Here's how the part is built. I have some questions about the finished solid (model axes, mm). Face numbers are marked on the shaded views. A direction names the side the tool comes from. Give positions to 0.01 mm unless a question says otherwise; leave off trailing zeros. Loops run counter-clockwise (first coordinate to the right, second up) from the corner with the lowest first, then second, coordinate; pieces in that order, holes last.
Q1. Suppose I cut it at A-A (z = 25.2). List the corners of the cut face in (x, y) for me, and give its area (3 significant figures).
Q2. Suppose I cut it at D-D (x = -8.25). List the corners of the cut face in (y, z) for me.
Q3. I'm going to push flat-ended pins straight in: P1, Ø5, axis at x = 12.5, y = -3, coming from the +Z side; P2, Ø3.5, axis at x = 10, y = 0.5, coming from the -Z side; P3, Ø4, axis at y = -4.5, z = 1, coming from the +X side. Where does each tip first touch, or does it pass through?
Q4. Suppose I cut it at B-B (x = 6.5). List the corners of the cut face in (y, z) for me.
Q5. For the marked faces 1, 2 and 3, which set-ups out of +Z, -Z, +X, -X, +Y, -Y let a thin tool reach every point of the face, with its end or its side?
Q6. I need wall thicknesses on probe 1 along Z at (x, y) = (7.3, 0); probe 2 along Z at (x, y) = (-5.75, 2); probe 3 along X at (y, z) = (-4, -2). Which ranges of each line are inside material? Lowest first, please.
Q7. Suppose I cut it at C-C (y = -4.5). List the corners of the cut face in (x, z) for me.
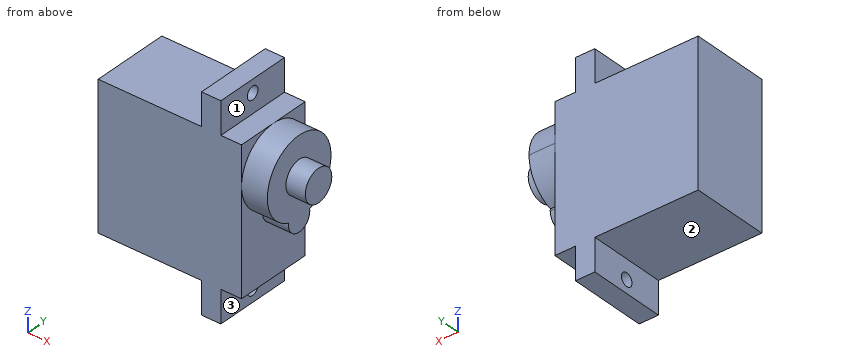
```python
from build123d import *

# Parameters (mm, degrees)
F1_DEPTH  = 22.2
F2_W      = 3
F2_H      = 12
F3_DEPTH  = 5
F4_W      = 3
F4_H      = 12
F5_DEPTH  = 5
F7_DEPTH  = 4
F8_R      = 2.5
F9_DEPTH  = 3
F10_R     = 1
F11_DEPTH = 25


with BuildPart() as f1:
    # F0 (on Top) → F1 (new body)
    with BuildSketch(Plane.XY):
        Polygon((-11.1, 6), (-11.1, 0), (-11.1, -6), (11.1, -6), (11.1, 0), (11.1, 6), align=None)
    extrude(amount=F1_DEPTH)

    # F2 (on face) → F3 (join)
    with BuildSketch(Plane.XY.offset(22.2)):
        with Locations((6.4, 0)):
            Rectangle(F2_W, F2_H)
    extrude(amount=F3_DEPTH)

    # F4 (on face) → F5 (join)
    with BuildSketch(Plane(origin=(0, 0, 0), x_dir=(1, 0, 0), z_dir=(0, 0, -1))):
        with Locations((6.4, 0)):
            Rectangle(F4_W, F4_H)
    extrude(amount=F5_DEPTH)

    # F6 (on face) → F7 (join)
    with BuildSketch(Plane.YZ.offset(11.1)):
        with BuildLine():
            ThreePointArc((1.9720265944, 10.5333333333), (4.8904069139, 12.7238066485), (6, 16.2))
            ThreePointArc((6, 16.2), (-3.4761933515, 21.0904069139), (-1.9720265944, 10.5333333333))
            ThreePointArc((-1.9720265944, 10.5333333333), (0, 12.2), (1.9720265944, 10.5333333333))
        make_face()
        with BuildLine():
            ThreePointArc((1.9720265944, 10.5333333333), (0, 12.2), (-1.9720265944, 10.5333333333))
            ThreePointArc((-1.9720265944, 10.5333333333), (0, 10.2), (1.9720265944, 10.5333333333))
        make_face()
        with BuildLine():
            ThreePointArc((1.9720265944, 10.5333333333), (0, 10.2), (-1.9720265944, 10.5333333333))
            ThreePointArc((-1.9720265944, 10.5333333333), (-0.1672525206, 8.2070056211), (2, 10.2))
            ThreePointArc((2, 10.2), (1.9929943789, 10.3672525206), (1.9720265944, 10.5333333333))
        make_face()
    extrude(amount=F7_DEPTH)

    # F8 (on face) → F9 (join)
    with BuildSketch(Plane.YZ.offset(15.1)):
        with Locations((0, 16.2)):
            Circle(F8_R)
    extrude(amount=F9_DEPTH)

    # F10 (on face) → F11 (cut)
    with BuildSketch(Plane(origin=(4.9, 0, 0), x_dir=(0, -1, 0), z_dir=(-1, 0, 0))):
        with Locations((0, 25.2)):
            Circle(F10_R)
        with Locations((0, -3)):
            Circle(F10_R)
    extrude(amount=-F11_DEPTH, mode=Mode.SUBTRACT)


solid = f1.part
```
Solutions:
1. outline: (4.9, -6) - (7.9, -6) - (7.9, -1) - (4.9, -1) - close; (4.9, 1) - (7.9, 1) - (7.9, 6) - (4.9, 6) - close
1. area: 30.0 mm2
2. outline: (-6, 0) - (6, 0) - (6, 22.2) - (-6, 22.2) - close
3. P1: stops at z = 22.2
3. P2: stops at z = 0
3. P3: stops at x = 11.1
4. outline: (-6, -5) - (6, -5) - (6, 27.2) - (-6, 27.2) - close; hole circle Ø2 at (0, -3); hole circle Ø2 at (0, 25.2)
5. face 1: +Z, +X, +Y, -Y
5. face 2: -Z, -X, +Y, -Y
5. face 3: -Z, +X, +Y, -Y
6. probe 1: z = -5 to -4, -2 to 24.2, 26.2 to 27.2
6. probe 2: z = 0 to 22.2
6. probe 3: x = 4.9 to 7.9
7. outline: (-11.1, 0) - (4.9, 0) - (4.9, -5) - (7.9, -5) - (7.9, 0) - (11.1, 0) - (11.1, 12.23) - (15.1, 12.23) - (15.1, 20.17) - (11.1, 20.17) - (11.1, 22.2) - (7.9, 22.2) - (7.9, 27.2) - (4.9, 27.2) - (4.9, 22.2) - (-11.1, 22.2) - close
